Read the model definition and answer for the solid it produces. Units are mm, in the model's axes. A direction names the side the tool comes from. Coordinates: 2 decimals unless noted, no trailing zeros. Loops run counter-clockwise (first coordinate to the right, second up) from the corner with the lowest first, then second, coordinate; pieces in that order, holes last. Notation, with made-up numbers: M 84.5,73 L 119.5,73 A18 ccw 119.5,90 Z; hole C -32,56 d8. An arc over 180 degrees is marked long. Use one line per item in the form item = value. Start each with the question number.
1. A flat-ended cylindrical pin translates along its axis: pin 1 (1 mm diameter, centred on x = -4.5, y = 4.5, fed in from +Z). Find the tip coordinate at first contact, or state that the pin passes through.
2. A tool of negligible diameter and unlimited length cuts with its end or side. For faces 1 (the flat face through (0, -33, 7)), 2 (the flat face through (0, -35, 6)), from which of +Z, -Z, +X, -X, +Y, -Y can it reach the whole face along a straight path? Write none if from no direction.
3. The part is cut by section C-C (x = -20). Give the vertices of the cut face in (y, z), plus the area to 3 significant figures.
4. The part is cut by section A-A (z = 4.75). Give the vertices of the cut face in (x, y), plus the area to 3 significant figures.
5. Find the intervals of material crossed by probe 1 along X at (y, z) = (17, 2.25); probe 2 along Y at (x, z) = (29, 2.5); probe 3 along Z at (x, y) = (-29, 22), in increasing order. Write a range as [from, to].
6. The part is cut by section B-B (y = 13.5). Give the vertices of the cut face in (x, z), plus the area to 3 significant figures.
7. For a pull along X with two mould halves and no side action, classify faces 3 (the flat face through (0, 0, 0)), 4 (the flat face through (-34, 0, 6)), 5 (the flat face through (32, 0, 7)) as released by +X, released by -X, zero draft, split by the parting line, or undercut.
from build123d import *

# Parameters (mm, degrees)
F0_W     = 68
F0_H     = 70
F0_W_2   = 64
F0_H_2   = 66
F1_DEPTH = 12
F2_R     = 0.5
F3_W     = 64
F3_H     = 2
F4_DEPTH = 66


with BuildPart() as f1:
    # F0 (on Top) → F1 (new body)
    with BuildSketch(Plane.XY):
        Rectangle(F0_W, F0_H)
        Rectangle(F0_W_2, F0_H_2, mode=Mode.SUBTRACT)
    extrude(amount=F1_DEPTH)

    # F2
    f2_edges = [f1.edges().sort_by_distance(p)[0] for p in [
        (-34, 0, 12),
        (0, -35, 12),
        (0, 35, 12),
        (34, 0, 12),
        (-32, 0, 12),
        (0, 33, 12),
        (32, 0, 12),
        (0, -33, 12),
    ]]
    fillet(f2_edges, radius=F2_R)

    # F3 (on face) → F4 (join, through all)
    with BuildSketch(Plane.XZ.offset(-33)):
        with Locations((0, 1)):
            Rectangle(F3_W, F3_H)
    extrude(amount=F4_DEPTH)


solid = f1.part
Computed values:
q1.pin_1 = 2
q2.face_1 = +Z
q2.face_2 = +Z, -Z, +X, -X, -Y
q3.outline = M -35,0 L 35,0 L 35,11.5 A0.5 ccw 34.5,12 L 33.5,12 A0.5 ccw 33,11.5 L 33,2 L -33,2 L -33,11.5 A0.5 ccw -33.5,12 L -34.5,12 A0.5 ccw -35,11.5 Z
q3.area = 180 mm²
q4.outline = M -34,-35 L 34,-35 L 34,35 L -34,35 Z; hole M -32,-33 L 32,-33 L 32,33 L -32,33 Z
q4.area = 536 mm²
q5.probe_1 = [-34, -32], [32, 34]
q5.probe_2 = [-35, -33], [33, 35]
q5.probe_3 = [0, 2]
q6.outline = M -34,0 L 34,0 L 34,11.5 A0.5 ccw 33.5,12 L 32.5,12 A0.5 ccw 32,11.5 L 32,2 L -32,2 L -32,11.5 A0.5 ccw -32.5,12 L -33.5,12 A0.5 ccw -34,11.5 Z
q6.area = 176 mm²
q7.face_3 = zero draft
q7.face_4 = released by -X
q7.face_5 = undercut
